from build123d import *

# Parameters (mm, degrees)
SKETCH1_W           = 22
SKETCH1_H           = 40
SKETCH1_R           = 2.125
BOSS_EXTRUDE1_DEPTH = 5
BOSS_EXTRUDE3_DEPTH = 40
FILLET1_R           = 2
SKETCH6_R           = 2.125
CUT_EXTRUDE1_DEPTH  = 7.086873748


with BuildPart() as part:
    # Sketch1 → Boss-Extrude1 (new body)
    with BuildSketch(Plane(origin=(0, 0, 0), x_dir=(1, 0, 0), z_dir=(0, 1, 0))):
        Rectangle(SKETCH1_W, SKETCH1_H)
        with Locations(Location((0, 15, 0), (0, 0, 270))):
            Circle(SKETCH1_R, mode=Mode.SUBTRACT)
        with Locations(Location((0, -15, 0), (0, 0, 270))):
            Circle(SKETCH1_R, mode=Mode.SUBTRACT)
    extrude(amount=BOSS_EXTRUDE1_DEPTH)

    # Sketch4 → Boss-Extrude3 (add)
    with BuildSketch(Plane(origin=(0, 0, -20), x_dir=(-1, 0, 0), z_dir=(0, 0, -1))):
        Polygon((-11, 5), (-12, 5), (-12, 8.5), (-15, 8.5), (-15, 0), (-11, 0), align=None)
        Polygon((11, 0), (11, 5), (12, 5), (12, 8.5), (15, 8.5), (15, 0), align=None)
    extrude(amount=-BOSS_EXTRUDE3_DEPTH)

    # Fillet1
    fillet1_edges = [part.edges().sort_by_distance(p)[0] for p in [
        (15, 0, 0),
        (15, 8.5, 0),
        (-15, 0, 0),
        (-15, 8.5, 0),
    ]]
    fillet(fillet1_edges, radius=FILLET1_R)

    # Sketch2 → Loft1 section 0
    with BuildSketch(Plane.XZ):
        with BuildLine():
            Line((-11, 0.105117767), (11, 6))
            Line((11, 6), (11, -2))
            Line((11, -2), (-11, -7.894882233))
            Line((-11, -7.894882233), (-11, 0.105117767))
        make_face()
    # Sketch5 → Loft1 section 1
    with BuildSketch(Plane(origin=(0, -20, 0), x_dir=(-1, 0, 0), z_dir=(0, -1, 0))):
        with BuildLine():
            Line((-11, 3), (-11, 11))
            Line((-11, 11), (11, 16.894882233))
            Line((11, 16.894882233), (11, 8.894882233))
            Line((11, 8.894882233), (-11, 3))
        make_face()
    loft()

    # Sketch6 → Cut-Extrude1 (cut)
    with BuildSketch(Plane(origin=(1.040309356, 1.747119317, -3.882487372), x_dir=(0.9714204714250083, -0.09740631922929449, 0.21645848717621435), z_dir=(-0.2373652621939752, -0.3986366483069059, 0.8858592184598079))):
        with Locations(Location((5.252708211, -11.411685947, 0), (0, 0, 90))):
            Circle(SKETCH6_R)
        with Locations(Location((-7.39453945, -12.762593713, 0), (0, 0, 90))):
            Circle(SKETCH6_R)
    extrude(amount=CUT_EXTRUDE1_DEPTH, mode=Mode.SUBTRACT)


solid = part.part
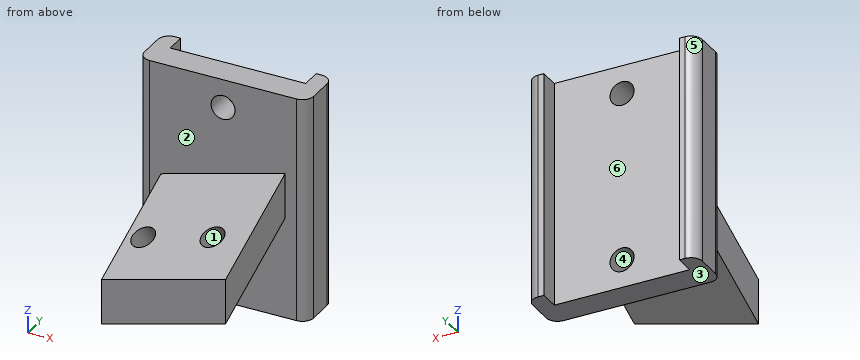
Design review of the part built by this model. Coordinates are the model's own, in mm. Face numbers are marked on the shaded views. A direction names the side the tool comes from. Give positions to 0.01 mm unless a question says otherwise; leave off trailing zeros. Order: outer loops, then holes, each group sorted by start corner. A loop starts at its lowest first (then second) coordinate and runs counter-clockwise, first axis right, second up. Notation, with made-up numbers: (-14.75, -32.5) - (-9.75, -32.5) arc R20 cw to (-9.75, -10.5) - close; hole circle Ø6 at (47, 60). An arc over 180 degrees is marked (long way). Write item = value, one per line. Start each with the question number.
Q1. We need section A-A on z = 15. State the section outline as (x, y) points (3 decimals).
Q2. Tool access review of the marked faces 4, 5 and 6: name each direction out of +Z, -Z, +X, -X, +Y, -Y from which nothing blocks a thin tool from reaching the whole face with its end or side.
Q3. Clearance check with flat-ended pins moving along their axes: pin 1 Ø7 at (x, z) = (0, 15) entering from -Y; pin 2 Ø8 at (y, z) = (-14, -1) entering from +X; pin 3 Ø3 at (y, z) = (-7, -12.5) entering from -X. State where each tip first meets the part, or that it passes through.
Q4. We need section C-C on z = -15. State how many separate pieces and enclosed holes the cut face has, plus the area to 3 significant figures.
Q5. We need section B-B on x = 11.5. State the section outline as (y, z) points, plus the area to 3 significant figures.
Q6. To check wall thickness, follow L1, parallel to X at y = 2.7, z = 15 (3 decimals); L2, parallel to X at y = -11.5, z = -5.5; L3, parallel to X at y = 6, z = -10. State the ranges of each line that lie inside material, in increasing order. Write a range as from..to.
Q7. Mouldability with a two-part tool opening along Z and no side actions: class the marked faces 1, 2 and 3 as released by +Z, released by -Z, zero draft, split by the parting line, or undercut.
Working result:
q1.outline = (-15, 2) arc R2 ccw to (-13, 0) - (-2.125, 0) - (-2.125, 5) - (-12, 5) - (-12, 8.5) - (-13, 8.5) arc R2 ccw to (-15, 6.5) - close; (2.125, 0) - (13, 0) arc R2 ccw to (15, 2) - (15, 6.5) arc R2 ccw to (13, 8.5) - (12, 8.5) - (12, 5) - (2.125, 5) - close
q2.face_4 = +Y
q2.face_5 = +Z, -Z, -X, +Y
q2.face_6 = +Z, -Z, +Y
q3.pin_1 = 0
q3.pin_2 = 11
q3.pin_3 = -11
q4.separate_pieces = 3
q4.enclosed_holes = 0
q4.area = 161 mm²
q5.outline = (0, -20) - (5, -20) - (5, 20) - (0, 20) - close
q5.area = 200 mm²
q6.L1 = -15..-2.125, 2.125..15
q6.L2 = -11..-9.73, -5.35..3.78, 7.18..11
q6.L3 = -15..-12, 12..15
q7.face_1 = undercut
q7.face_2 = zero draft
q7.face_3 = released by -Z
